Here's how the part is built. I have some questions about the finished solid (model axes, mm). A direction names the side the tool comes from. Round coordinates to 2 decimals unless told otherwise and drop trailing zeros. Order: outer loops, then holes, each group sorted by start corner. A loop starts at its lowest first (then second) coordinate and runs counter-clockwise, first axis right, second up. Notation, with made-up numbers: (36.5, 51) -> (85.5, 51) arc R18 ccw to (85.5, 70) -> close; hole circle Ø11 at (44.25, 41.25). An arc over 180 degrees is marked (long way). Answer in a Markdown table with one row per item.
```python
from build123d import *

# Parameters (mm, degrees)
SKETCH1_R               = 15
BOSS_EXTRUDE1_DEPTH     = 5
SKETCH2_R               = 10
BOSS_EXTRUDE2_DEPTH     = 145
SKETCH3_W               = 15
SKETCH3_H               = 10
BOSS_EXTRUDE3_DEPTH     = 20
CUT_EXTRUDE1_DEPTH      = 153.069063257
CUT_EXTRUDE1_DEPTH_BACK = 153.069063257
SKETCH4_R               = 5
CUT_EXTRUDE2_DEPTH      = 172.31841699
CUT_EXTRUDE2_DEPTH_BACK = 15
SKETCH5_W               = 15
SKETCH5_H               = 7
FILLET1_R               = 7.5


with BuildPart() as part:
    # Sketch1 → Boss-Extrude1 (new body)
    with BuildSketch(Plane(origin=(0, 0, 0), x_dir=(1, 0, 0), z_dir=(0, 1, 0))):
        with Locations(Location((0, 0, 0), (0, 0, 270))):
            Circle(SKETCH1_R)
    extrude(amount=BOSS_EXTRUDE1_DEPTH)

    # Sketch2 → Boss-Extrude2 (add)
    with BuildSketch(Plane(origin=(0, 5, 0), x_dir=(1, 0, 0), z_dir=(0, 1, 0))):
        with Locations(Location((0, 0, 0), (0, 0, 270))):
            Circle(SKETCH2_R)
    extrude(amount=BOSS_EXTRUDE2_DEPTH)

    # Sketch3 → Boss-Extrude3 (add)
    with BuildSketch(Plane.XZ):
        Rectangle(SKETCH3_W, SKETCH3_H)
    extrude(amount=BOSS_EXTRUDE3_DEPTH)

    # Sketch4 → Cut-Extrude1 (cut, two sides: drawn at the far end of the back side and taken through both)
    with BuildSketch(Plane.XY.offset(5).offset(-CUT_EXTRUDE1_DEPTH_BACK)):
        with Locations((0, -12.5)):
            Circle(SKETCH4_R)
    extrude(amount=CUT_EXTRUDE1_DEPTH + CUT_EXTRUDE1_DEPTH_BACK, mode=Mode.SUBTRACT)

    # Sketch5 → Cut-Extrude2 (cut, two sides: drawn at the far end of the back side and taken through both)
    with BuildSketch(Plane.XZ.offset(20).offset(-CUT_EXTRUDE2_DEPTH_BACK)):
        Rectangle(SKETCH5_W, SKETCH5_H)
    extrude(amount=CUT_EXTRUDE2_DEPTH + CUT_EXTRUDE2_DEPTH_BACK, mode=Mode.SUBTRACT)

    # Fillet1
    fillet1_edges = [part.edges().sort_by_distance(p)[0] for p in [
        (7.5, -20, 4.25),
        (7.5, -20, -4.25),
        (-7.5, -20, 4.25),
        (-7.5, -20, -4.25),
    ]]
    fillet(fillet1_edges, radius=FILLET1_R - 0.0001)  # a hair under: the kernel refuses the full size


solid = part.part
```
1. Suppose I cut it at A-A on x = -2.25. Write out the boundary of the cut face in (y, z).
Numbers:
| item | result |
|---|---|
| outline | (-19.65, -5) -> (-16.97, -5) -> (-16.97, -3.5) -> (-19.65, -3.5) -> close; (-19.65, 3.5) -> (-16.97, 3.5) -> (-16.97, 5) -> (-19.65, 5) -> close; (-8.03, -5) -> (0, -5) -> (0, -14.83) -> (5, -14.83) -> (5, -9.74) -> (150, -9.74) -> (150, 9.74) -> (5, 9.74) -> (5, 14.83) -> (0, 14.83) -> (0, 5) -> (-8.03, 5) -> (-8.03, 3.5) -> (-5, 3.5) -> (-5, -3.5) -> (-8.03, -3.5) -> close |
2. We'd pull the mould along Y, two halves only. Please class faces 1 (the face through (-1.8, -7.6, 5)), 2 (the face through (0, 0, 6)), 3 (the face through (2.688, -8.284, -4.261)): released by +Y, released by -Y, zero draft, split by the parting line, or undercut.
Numbers:
| item | result |
|---|---|
| face 1 | zero draft |
| face 2 | released by -Y |
| face 3 | undercut |
3. Suppose I cut it at B-B on z = 0. Write out the boundary of the cut face in (x, y).
Numbers:
| item | result |
|---|---|
| outline | (-15, 0) -> (-7.5, 0) -> (-7.5, -5) -> (7.5, -5) -> (7.5, 0) -> (15, 0) -> (15, 5) -> (10, 5) -> (10, 150) -> (-10, 150) -> (-10, 5) -> (-15, 5) -> close |
4. Suppose I cut it at D-D on z = -8.25. Write out the boundary of the cut face in (x, y), then the cut area to 3 significant figures.
Numbers:
| item | result |
|---|---|
| outline | (-12.53, 0) -> (12.53, 0) -> (12.53, 5) -> (5.65, 5) -> (5.65, 150) -> (-5.65, 150) -> (-5.65, 5) -> (-12.53, 5) -> close |
| area | 1,760 mm2 |
5. Please list where these lines run through material, in increasing order: line 1 along Y through (x, z) = (0, 4.7); line 2 along X through (y, z) = (-12.5, 4.2); line 3 along Y through (x, z) = (-6.75, -7).
Numbers:
| item | result |
|---|---|
| line 1 | y = -20 to -17.5, -7.5 to 150 |
| line 2 | x = -7.5 to -5, 5 to 7.5 |
| line 3 | y = 0 to 150 |
6. For faces 4 (the face through (-10, 5, 3)), 5 (the face through (-1.8, -7.6, -5)), 6 (the face through (7.5, -3, 0)), 7 (the face through (-7.5, -3, 0)), which set-ups out of +Z, -Z, +X, -X, +Y, -Y let a thin tool reach every point of the face, with its end or its side?
Numbers:
| item | result |
|---|---|
| face 4 | +Y |
| face 5 | -Z, +X, -X, -Y |
| face 6 | +Z, -Z, +X, -Y |
| face 7 | +Z, -Z, -X, -Y |
7. For pin 1 Ø6 at (x, y) = (9, 7) entering from +Z; pin 2 Ø9 at (x, y) = (0, -12.5) entering from +Z; pin 3 Ø3 at (x, y) = (7, 114) entering from -Z; pin 4 Ø11.5 at (x, y) = (0, -12.5) entering from +Z, each with a flat end and sliding along its axis, tell me the tip position at first contact or that it passes through.
Numbers:
| item | result |
|---|---|
| pin 1 | stops at z = 13.39 |
| pin 2 | passes through |
| pin 3 | stops at z = -8.35 |
| pin 4 | stops at z = 5 |
8. Suppose I cut it at C-C on y = 81. Write out the boundary of the cut face in (x, z).
Numbers:
| item | result |
|---|---|
| outline | circle Ø20 at (0, 0) |
